The figure shows three views and two pictorial views of one solid part (mm, origin at its lowest corner). Answer the questions. A direction names the side the tool comes from. Give positions to 0.01 mm unless a question says otherwise; leave off trailing zeros. Loops run counter-clockwise (first coordinate to the right, second up) from the corner with the lowest first, then second, coordinate; pieces in that order, holes last. Notation, with made-up numbers: (30.25, -16.75) - (41.25, -16.75) arc R18 ccw to (41.25, -0.75) - close; hole circle Ø2 at (32.25, -5). An arc over 180 degrees is marked (long way). Use a Markdown table: item, result. Add a question column.
Item 1: A cutting plane is placed at C-C (z = 13). Determine the outline of the cut face in (x, y) (1 decimal).
Item 2: Each of these flat-tipped pins is pushed along its axis until it touches: P1, Ø5.5, axis at x = 19.5, y = 5, coming from the +Z side; P2, Ø3, axis at y = 13, z = 16.5, coming from the -X side; P3, Ø14.5, axis at x = 22, z = 15.5, coming from the +Y side; P4, Ø0.9, axis at x = 2, z = 24, coming from the -Y side. Where does it stop, or does it pass through?
Item 3: Consider probe 1 along Y at (x, z) = (24.25, 3.5); probe 2 along Y at (x, z) = (7.5, 13); probe 3 along Z at (x, y) = (14.5, 17). Determine where each line is inside the solid, lowest interval first. Write a range as [from, to].
Item 4: A cutting plane is placed at D-D (x = 8). Determine the outline of the cut face in (y, z), plus the area to 3 significant figures.
Item 5: Which of the six approach directions +Z, -Z, +X, -X, +Y, -Y give full straight-line access (tool end or side, diameter ignored) to the marked faces 1, 2, 3, 4 and 5?
Item 6: A cutting plane is placed at B-B (y = 5). Determine the outline of the cut face in (x, z), plus the area to 3 significant figures.
Item 7: A cutting plane is placed at A-A (x = 5). Determine the outline of the cut face in (y, z).
Item 8: For a pull along Z with two mould halves and no side action, classify the marked faces 6, 7 and 8 as +Z half, -Z half, draft (parallel to the pull), parting line (faces both ways), or undercut.
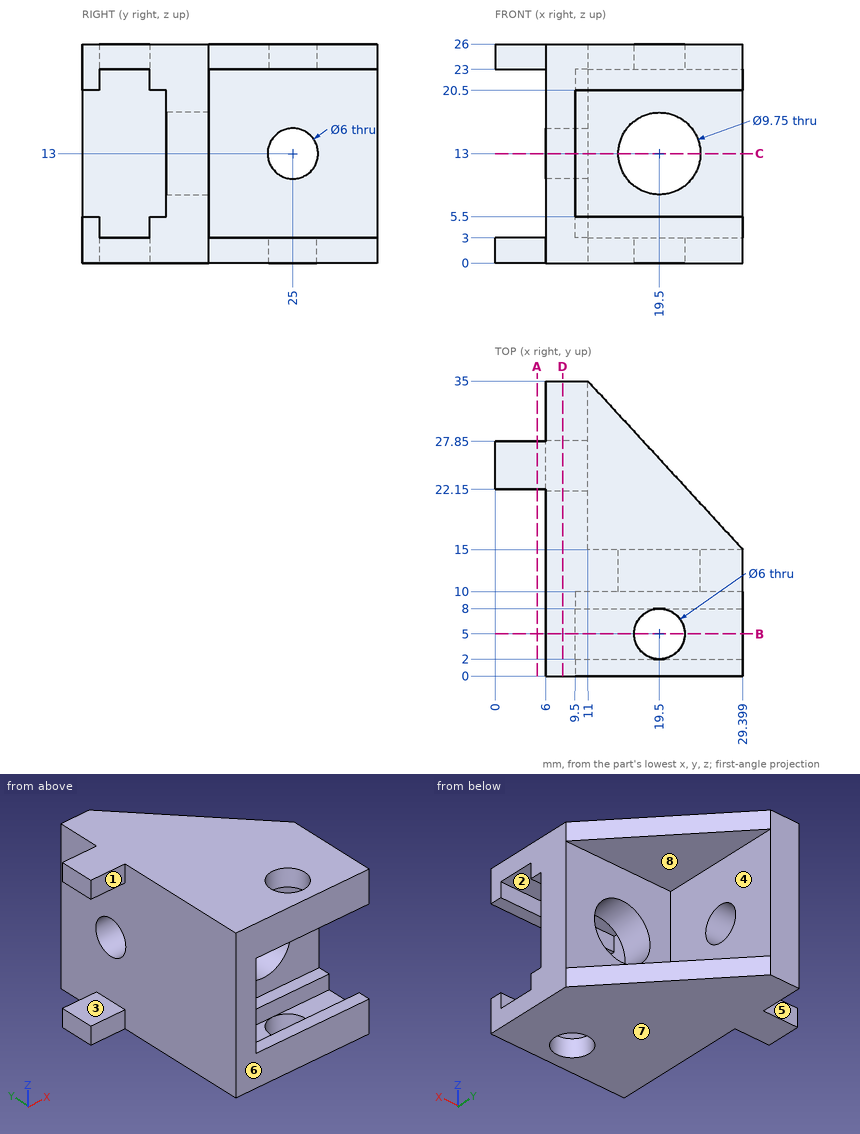
Geometry says:
| question | item | result |
|---|---|---|
| 1 | outline | (6, 0) - (9.5, 0) - (9.5, 10) - (14.6, 10) - (14.6, 15) - (11, 15) - (11, 22) - (6, 22) - close; (6, 28) - (11, 28) - (11, 35) - (6, 35) - close; (24.4, 10) - (29.4, 10) - (29.4, 15) - (24.4, 15) - close |
| 2 | P1 | through |
| 2 | P2 | x = 6 |
| 2 | P3 | y = 15 |
| 2 | P4 | y = 22.15 |
| 3 | probe 1 | [0, 2], [8, 15] |
| 3 | probe 2 | [0, 22], [28, 35] |
| 3 | probe 3 | [0, 3], [23, 26] |
| 4 | outline | (0, 0) - (35, 0) - (35, 26) - (0, 26) - close; hole circle Ø6 at (25, 13) |
| 4 | area | 882 mm² |
| 5 | face 1 | +Z, -Z, -X, -Y |
| 5 | face 2 | +X |
| 5 | face 3 | -X, +Y, -Y |
| 5 | face 4 | +X, +Y |
| 5 | face 5 | +Z, -Z, -X, +Y |
| 6 | outline | (6, 0) - (16.5, 0) - (16.5, 3) - (9.5, 3) - (9.5, 23) - (16.5, 23) - (16.5, 26) - (6, 26) - close; (22.5, 0) - (29.4, 0) - (29.4, 3) - (22.5, 3) - close; (22.5, 23) - (29.4, 23) - (29.4, 26) - (22.5, 26) - close |
| 6 | area | 174 mm² |
| 7 | outline | (22.15, 0) - (27.85, 0) - (27.85, 3) - (22.15, 3) - close; (22.15, 23) - (27.85, 23) - (27.85, 26) - (22.15, 26) - close |
| 8 | face 6 | draft |
| 8 | face 7 | -Z half |
| 8 | face 8 | undercut |
